The figure shows three views and two pictorial views of one solid part (mm, origin at its lowest corner). Answer the questions. A direction names the side the tool comes from. Coordinates: 2 decimals unless noted, no trailing zeros. Order: outer loops, then holes, each group sorted by start corner. A loop starts at its lowest first (then second) coordinate and runs counter-clockwise, first axis right, second up. Notation, with made-up numbers: M 42,58 L 96,58 A32 ccw 96,89 Z; hole C 3.5,56 d5. An arc over 180 degrees is marked long. Write item = value, one per line. Start each with the question number.
Q1. Find section C-C on z = 190.5. Give the number of separate pieces and of enclosed holes in the cut face, and give its area (3 significant figures).
Q2. Find section B-B on y = 849. Give the vertices of the cut face in (x, z).
Q3. A tool of negligible diameter and unlimited length cuts with its end or side. For the marked faces 4 and 5, from which of +Z, -Z, +X, -X, +Y, -Y can it reach the whole face along a straight path? Write none if from no direction.
Q4. Straight lines are drawn through the part: line 1 along Z through (x, y) = (1016, 997); line 2 along X through (y, z) = (466.5, 157); line 3 along Y through (x, z) = (155, 265). For each, find the intervals that lie inside material, in ascending order.
Q5. Find section A-A on x = 929.5. Give the vertices of the cut face in (y, z).
Q6. Find section D-D on z = 354.5. Give the vertices of the cut face in (x, y), and give its area (3 significant figures).
Q7. Determine the mould class of the marked faces 1, 2 and 3 for opening direction X: released by +X, released by -X, zero draft, split by the parting line, or undercut.
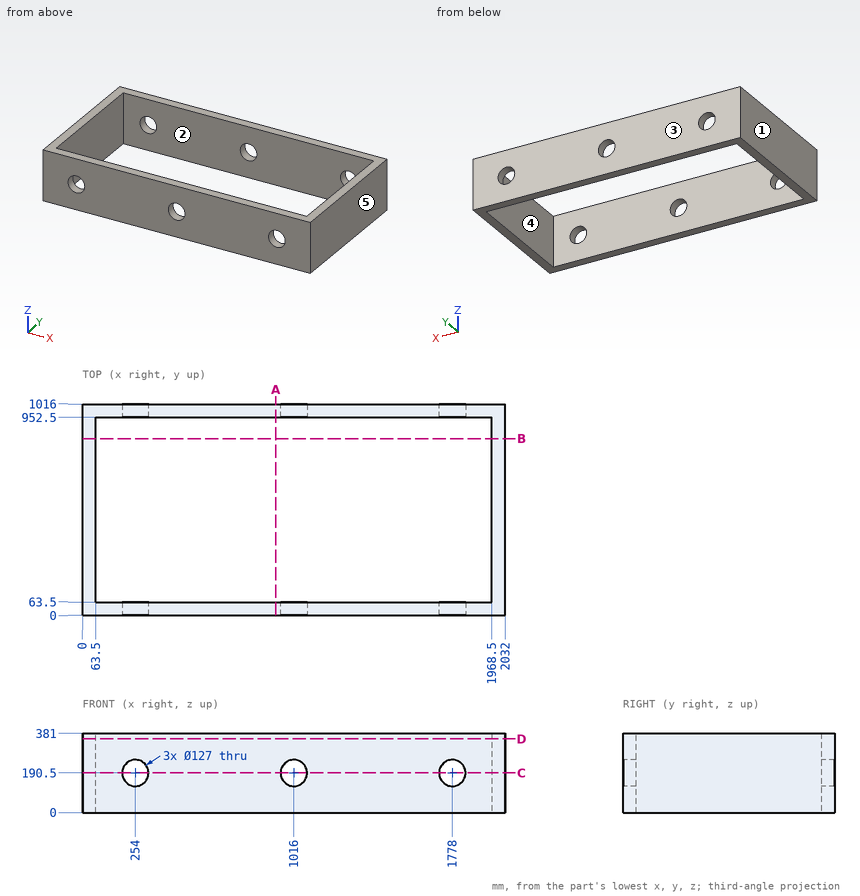
Findings below:
q1.separate_pieces = 6
q1.enclosed_holes = 0
q1.area = 323,000 mm^2
q2.outline = M 0,0 L 63.5,0 L 63.5,381 L 0,381 Z; M 1968.5,0 L 2032,0 L 2032,381 L 1968.5,381 Z
q3.face_4 = +Z, -Z
q3.face_5 = +Z, -Z, +X, +Y, -Y
q4.line_1 = 0 to 127, 254 to 381
q4.line_2 = 0 to 63.5, 1968.5 to 2032
q4.line_3 = 0 to 63.5, 952.5 to 1016
q5.outline = M 0,0 L 63.5,0 L 63.5,381 L 0,381 Z; M 952.5,0 L 1016,0 L 1016,381 L 952.5,381 Z
q6.outline = M 0,0 L 2032,0 L 2032,1016 L 0,1016 Z; hole M 63.5,63.5 L 1968.5,63.5 L 1968.5,952.5 L 63.5,952.5 Z
q6.area = 371,000 mm^2
q7.face_1 = released by -X
q7.face_2 = undercut
q7.face_3 = zero draft
